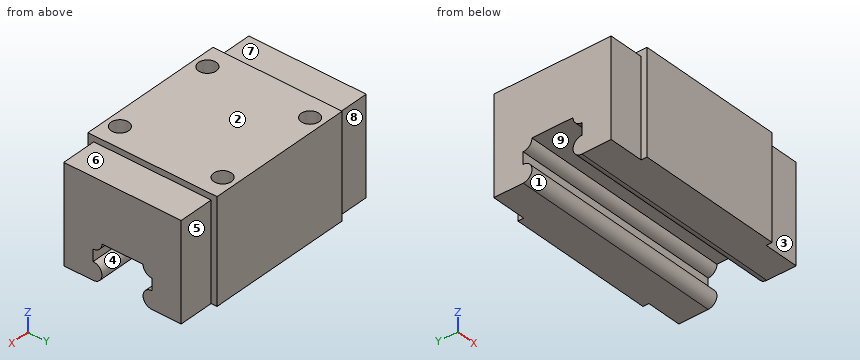
from build123d import *

# Parameters (mm, degrees)
F1_DEPTH  = 74
F2_W      = 12
F2_H      = 44
F3_DEPTH  = 2
F4_W      = 12
F4_H      = 2
F5_DEPTH  = 25
F7_DEPTH  = 8
F8_W      = 50
F8_H      = 44
F8_R      = 3
F9_DEPTH  = 10
F10_W     = 12
F10_H     = 40
F11_DEPTH = 10


with BuildPart() as f1:
    # F0 (on Right) → F1 (new body)
    with BuildSketch(Plane.YZ):
        with BuildLine():
            ThreePointArc((-26.041336, 5), (-23.041336, 8), (-26.041336, 11))
            Line((-26.041336, 11), (-26.041336, 15))
            ThreePointArc((-26.041336, 15), (-23.920016, 15.87868), (-23.041336, 18))
            Line((-23.041336, 18), (-9.041336, 18))
            ThreePointArc((-9.041336, 18), (-8.162657, 15.87868), (-6.041336, 15))
            Line((-6.041336, 15), (-6.041336, 11))
            ThreePointArc((-6.041336, 11), (-9.041336, 8), (-6.041336, 5))
            Line((-6.041336, 5), (5.958664, 5))
            Line((5.958664, 5), (5.958664, 30))
            Line((5.958664, 30), (-38.041336, 30))
            Line((-38.041336, 30), (-38.041336, 5))
            Line((-38.041336, 5), (-26.041336, 5))
        make_face()
    extrude(amount=F1_DEPTH)

    # F2 (on face) → F3 (cut)
    with BuildSketch(Plane.XY.offset(30)):
        with Locations((68, -16.041336)):
            Rectangle(F2_W, F2_H)
        with Locations((6, -16.041336)):
            Rectangle(F2_W, F2_H)
    extrude(amount=-F3_DEPTH, mode=Mode.SUBTRACT)

    # F4 (on face) → F5 (cut)
    with BuildSketch(Plane.XY.offset(30)):
        with Locations((6, 4.958664)):
            Rectangle(F4_W, F4_H)
        with Locations((6, -37.041336)):
            Rectangle(F4_W, F4_H)
        with Locations((68, -37.041336)):
            Rectangle(F4_W, F4_H)
        with Locations((68, 4.958664)):
            Rectangle(F4_W, F4_H)
    extrude(amount=-F5_DEPTH, mode=Mode.SUBTRACT)

    # F6 (on face) → F7 (cut)
    with BuildSketch(Plane.XY.offset(30)):
        with BuildLine():
            ThreePointArc((22.5, 1.458664), (17.37868, 3.579984), (19.5, -1.541336))
            ThreePointArc((19.5, -1.541336), (21.62132, -0.662657), (22.5, 1.458664))
        make_face()
        with BuildLine():
            ThreePointArc((51.5, 1.458664), (52.37868, -0.662657), (54.5, -1.541336))
            ThreePointArc((54.5, -1.541336), (56.62132, -0.662657), (57.5, 1.458664))
            ThreePointArc((57.5, 1.458664), (54.5, 4.458664), (51.5, 1.458664))
        make_face()
        with BuildLine():
            ThreePointArc((54.5, -30.541336), (52.37868, -31.420016), (51.5, -33.541336))
            ThreePointArc((51.5, -33.541336), (54.5, -36.541336), (57.5, -33.541336))
            ThreePointArc((57.5, -33.541336), (56.62132, -31.420016), (54.5, -30.541336))
        make_face()
        with BuildLine():
            ThreePointArc((19.5, -30.541336), (17.37868, -35.662657), (22.5, -33.541336))
            ThreePointArc((22.5, -33.541336), (21.62132, -31.420016), (19.5, -30.541336))
        make_face()
    extrude(amount=-F7_DEPTH, mode=Mode.SUBTRACT)

    # F8 (on face) → F9 (join)
    with BuildSketch(Plane.XY.offset(30)):
        with Locations((37, -16.041336)):
            Rectangle(F8_W, F8_H)
        with Locations((19.5, -33.541336)):
            Circle(F8_R, mode=Mode.SUBTRACT)
        with Locations((54.5, -33.541336)):
            Circle(F8_R, mode=Mode.SUBTRACT)
        with Locations((19.5, 1.458664)):
            Circle(F8_R, mode=Mode.SUBTRACT)
        with Locations((54.5, 1.458664)):
            Circle(F8_R, mode=Mode.SUBTRACT)
    extrude(amount=F9_DEPTH)

    # F10 (on face) → F11 (join)
    with BuildSketch(Plane.XY.offset(28)):
        with Locations((6, -16.041336)):
            Rectangle(F10_W, F10_H)
        with Locations((68, -16.041336)):
            Rectangle(F10_W, F10_H)
    extrude(amount=F11_DEPTH)


solid = f1.part
Verification items for the finished model (mm, model axes). Face numbers are marked on the shaded views. A direction names the side the tool comes from. Coordinates: 2 decimals unless noted, no trailing zeros. Write each loop counter-clockwise with the first axis right and the second up, starting at its lowest first coordinate (ties: lowest second). Pieces come first, ordered by that corner, then holes. Notation, with made-up numbers: M -40,80.5 L -9,80.5 A31 ccw -9,119.5 Z; hole C 19.25,-39.75 d10. An arc over 180 degrees is marked long. Use a Markdown table: item, result.
Q1. Go/stop test with flat-tipped pins: P1, Ø1.8, axis at x = 53, y = 1, coming from the +Z side; P2, Ø9.5, axis at x = 70.5, z = 19.5, coming from the +Y side; P3, Ø3.5, axis at x = 4.5, z = 23.5, coming from the -Y side. Record where each tip stops, or that it passes through.
Reply:
| item | result |
|---|---|
| P1 | stops at z = 22 |
| P2 | stops at y = 3.96 |
| P3 | stops at y = -36.04 |
Q2. Sectioned sample at B-B, the plane y = -29. Record the boundary of the cut face in (x, z).
Reply:
| item | result |
|---|---|
| outline | M 0,5 L 74,5 L 74,38 L 62,38 L 62,40 L 12,40 L 12,38 L 0,38 Z |
Q3. Draft check along Y on the marked faces 1, 2, 3 and 4. Enter one of: +Y half, -Y half, draft (parallel to the pull), parting line (faces both ways), or undercut.
Reply:
| item | result |
|---|---|
| face 1 | undercut |
| face 2 | draft |
| face 3 | -Y half |
| face 4 | undercut |
Q4. Sectioned sample at D-D, the plane z = 21. Record the boundary of the cut face in (x, y).
Reply:
| item | result |
|---|---|
| outline | M 0,-36.04 L 12,-36.04 L 12,-38.04 L 62,-38.04 L 62,-36.04 L 74,-36.04 L 74,3.96 L 62,3.96 L 62,5.96 L 12,5.96 L 12,3.96 L 0,3.96 Z |
Q5. Thickness scan on line 1 (Y direction, x = 19.5, z = 26.5); line 2 (Y direction, x = 19, z = 34); line 3 (X direction, y = 0, z = 24). Record the ranges inside material, lowest first.
Reply:
| item | result |
|---|---|
| line 1 | y = -38.04 to -36.54, -30.54 to -1.54, 4.46 to 5.96 |
| line 2 | y = -38.04 to -36.5, -30.58 to -1.5, 4.42 to 5.96 |
| line 3 | x = 0 to 16.88, 22.12 to 51.88, 57.12 to 74 |
Q6. Sectioned sample at C-C, the plane x = 6. Record the boundary of the cut face in (y, z).
Reply:
| item | result |
|---|---|
| outline | M -36.04,5 L -26.04,5 A3 ccw -26.04,11 L -26.04,15 A3 ccw -23.04,18 L -9.04,18 A3 ccw -6.04,15 L -6.04,11 A3 ccw -6.04,5 L 3.96,5 L 3.96,38 L -36.04,38 Z |
Q7. Set-up check for the marked faces 5, 6, 7, 8 and 9: record each of +Z, -Z, +X, -X, +Y, -Y from which the full face is reachable in a straight line by a thin tool's end or side.
Reply:
| item | result |
|---|---|
| face 5 | +Z, -Z, +X, +Y |
| face 6 | +Z, +X, +Y, -Y |
| face 7 | +Z, -X, +Y, -Y |
| face 8 | +Z, -Z, -X, +Y |
| face 9 | -Z, +X, -X |
Q8. Sectioned sample at A-A, the plane z = 8. Record the boundary of the cut face in (x, y).
Reply:
| item | result |
|---|---|
| outline | M 0,-36.04 L 12,-36.04 L 12,-38.04 L 62,-38.04 L 62,-36.04 L 74,-36.04 L 74,-23.04 L 0,-23.04 Z; M 0,-9.04 L 74,-9.04 L 74,3.96 L 62,3.96 L 62,5.96 L 12,5.96 L 12,3.96 L 0,3.96 Z |
